from build123d import *

# Parameters (mm, degrees)
SKETCH2_R           = 1.905
BOSS_EXTRUDE5_DEPTH = 30.48
SKETCH3_W           = 77.139019834
SKETCH3_H           = 253.707230816
CUT_EXTRUDE1_DEPTH  = 20.32


with BuildPart() as part:
    # Sketch2 → Boss-Extrude5 (new body)
    with BuildSketch(Plane(origin=(0, 6.35, 0), x_dir=(1, 0, 0), z_dir=(0, 1, 0))):
        Polygon((37.877734137, 124.478458264), (104.775, 124.478458264), (104.775, 118.128458264), (111.125, 118.128458264), (111.125, 124.478458264), (117.475, 124.478458264), (117.475, 111.778458264), (111.125, 111.778458264), (111.125, 105.428458264), (117.475, 105.428458264), (117.427603838, 19.255527471), (111.125, 19.255527471), (111.125, 12.7), (117.427603838, 12.7), (117.475, -12.7), (111.125, -12.7), (111.125, -19.05), (117.475, -19.05), (117.475, -117.410242597), (111.125, -117.410242597), (111.125, -123.760242597), (117.475, -123.760242597), (117.475, -136.460242597), (111.125, -136.460242597), (111.125, -130.101785028), (104.775, -130.101785028), (104.775, -136.460242597), (37.598341682, -136.460242597), (37.598341682, -123.760242597), (104.775, -123.760242597), (104.775, -111.031020805), (104.775, -24.950677477), (104.775, 19.255527471), (104.775, 25.571960959), (104.775, 99.037268217), (104.775, 105.428458264), (104.775, 111.778458264), (37.877734137, 111.778458264), align=None)
        with Locations((45.623485648, -130.101785028)):
            Circle(SKETCH2_R, mode=Mode.SUBTRACT)
        with Locations((47.180468273, 118.128458264)):
            Circle(SKETCH2_R, mode=Mode.SUBTRACT)
    extrude(amount=BOSS_EXTRUDE5_DEPTH)

    # Sketch3 → Cut-Extrude1 (cut)
    with BuildSketch(Plane(origin=(0, 36.83, 0), x_dir=(1, 0, 0), z_dir=(0, 1, 0))):
        with Locations((72.277192216, -6.116117848)):
            Rectangle(SKETCH3_W, SKETCH3_H)
    extrude(amount=-CUT_EXTRUDE1_DEPTH, mode=Mode.SUBTRACT)


solid = part.part
Check sheet for the modelled part. Datum: model origin and axes. Units: mm. A direction names the side the tool comes from. Round coordinates to 2 decimals unless told otherwise and drop trailing zeros. Loops run counter-clockwise (first coordinate to the right, second up) from the corner with the lowest first, then second, coordinate; pieces in that order, holes last. Notation, with made-up numbers: (3.25, -17) -> (62.25, -17) arc R13 ccw to (62.25, -8) -> close; hole circle Ø10 at (4.25, -32). An arc over 180 degrees is marked (long way). Put each result on its own line as item: value. Start each with the question number.
1. Section check B-B (x = 96.5). Enter the section's corners in (y, z).
2. Draft check along Z on faces 1 (the face through (114, 21, 19.05)), 2 (the face through (114, 21, 136.46)), 3 (the face through (111.125, 21, -121)), 4 (the face through (111.125, 21, -16)). Enter one of: +Z half, -Z half, draft (parallel to the pull), parting line (faces both ways), or undercut.
3. Access from +Z, -Z, +X, -X, +Y, -Y to the whole of each face (thin tool, end or side, straight path). Record for faces 5 (the face through (109, 12, 130.102)), 6 (the face through (114, 21, 12.7)), 7 (the face through (104.775, 11, 4)), 8 (the face through (104.775, 18, -122)).
4. Scan lines: probe 1 along Z at (x, y) = (45, 22.5); probe 2 along Z at (x, y) = (101, 14); probe 3 along X at (y, z) = (21, -25). Record each from-to range of solid material in increasing order.
5. Section check D-D (z = 102.5). Enter the section's corners in (x, y) (3 decimals).
6. Gauge pin test, flat ends, axial feed: pin 1 (12 mm diameter, centred on y = 31.5, z = -70.5, fed in from -X); pin 2 (5 mm diameter, centred on y = 12, z = -29, fed in from -X) (3 decimals); pin 3 (6 mm diameter, centred on y = 22, z = -16, fed in from +X) (3 decimals). Record the tip position at first contact, or that the pin passes through.
7. Section check A-A (y = 21). Give the number of separate pieces and of enclosed holes in the cut face, plus the area to 3 significant figures.
Findings:
1. outline: (6.35, -124.48) -> (36.83, -124.48) -> (36.83, -120.74) -> (16.51, -120.74) -> (16.51, -111.78) -> (6.35, -111.78) -> close; (6.35, 123.76) -> (16.51, 123.76) -> (16.51, 132.97) -> (36.83, 132.97) -> (36.83, 136.46) -> (6.35, 136.46) -> close
2. face 1: undercut
2. face 2: +Z half
2. face 3: draft
2. face 4: undercut
3. face 5: +Z, +Y, -Y
3. face 6: +X, +Y, -Y
3. face 7: -X, +Y, -Y
3. face 8: -Z, +Y, -Y
4. probe 1: z = -124.48 to -120.74, 132.97 to 136.46
4. probe 2: z = -124.48 to -111.78, 123.76 to 136.46
4. probe 3: x = 110.85 to 117.43
5. outline: (104.775, 6.35) -> (117.475, 6.35) -> (117.475, 36.83) -> (110.847, 36.83) -> (110.847, 16.51) -> (104.775, 16.51) -> close
6. pin 1: stops at x = 110.85
6. pin 2: stops at x = 104.775
6. pin 3: stops at x = 111.125
7. separate pieces: 3
7. enclosed holes: 0
7. area: 2,050 mm^2
